Autodesk Inventor part; units mm, degrees
ref_plane "YZ Plane" through (0, 0, 0) normal (1, 0, 0) x (0, 1, 0)
ref_plane "XZ Plane" through (0, 0, 0) normal (0, 1, 0) x (-1, 0, 0)
ref_plane "XY Plane" through (0, 0, 0) normal (0, 0, 1) x (1, 0, 0)
sketch "Sketch1" plane through (0, 0, 0) normal (0, 0, 1) x (1, 0, 0)
  circle A0 centre (0, 0) radius 45
  circle A1 centre (0, 0) radius 10
  dimension "d0" = 90
  dimension "d1" = 20
extrude "Extrusion1" add sketch "Sketch1" along normal blind 10
hole "Hole1" at (0, 0, 0) direction (0, 0, 1) diameter 30 depth 4
sketch "Sketch2" plane through (0, 0, 0) normal (0, 0, -1) x (-1, 0, 0)
  circle A0 centre (0, 35) radius 3.6674
  point P0 (0, 0)
  dimension "d15" = 35
hole "Hole2" at (0, 35, 0) direction (0, 0, 1) diameter 6.6 end through all counterbore diameter 12 counterbore depth 2
chamfer "Chamfer1" distance 4 angle 45 1 edges at (0, 31.7, 10)
pattern_circular "Circular Pattern1" count 5 over 360 about axis through (0, 0, 0) along (0, 0, 1) of "Hole2", "Chamfer1"
properties part number "342-08" material "Titanium"
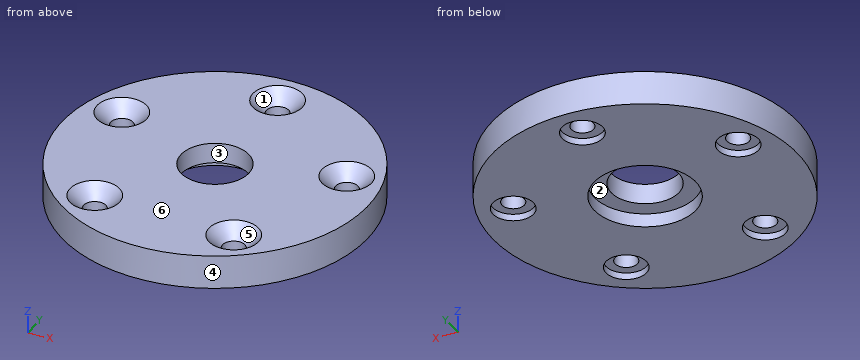
Verification items for the finished model (mm, model axes). Face numbers are marked on the shaded views. A direction names the side the tool comes from. Coordinates: 2 decimals unless noted, no trailing zeros. Order: outer loops, then holes, each group sorted by start corner. A loop starts at its lowest first (then second) coordinate and runs counter-clockwise, first axis right, second up. Notation, with made-up numbers: M 83,60 L 100,60 A36 ccw 100,99 Z; hole C 5,38.5 d1. An arc over 180 degrees is marked long. One line per item, written item: value. Start each with the question number.
Item 1: Sectioned sample at B-B (y = 0). Enter the section's corners in (x, z).
Item 2: Access from +Z, -Z, +X, -X, +Y, -Y to the whole of each face (thin tool, end or side, straight path). Record for the marked faces 1 and 2.
Item 3: Gauge pin test, flat ends, axial feed: pin 1 (6 mm diameter, centred on x = 35.5, y = 9.5, fed in from -Z); pin 2 (7 mm diameter, centred on x = -20.57, y = -28.32, fed in from +Z); pin 3 (5 mm diameter, centred on y = -30.5, z = 2, fed in from -X). Record the tip position at first contact, or that the pin passes through.
Item 4: Sectioned sample at D-D (y = -17). Enter the section's corners in (x, z).
Item 5: Mould release check, pull along X, two halves, no side actions. Record for the marked faces 3, 4, 5 and 6: released by +X, released by -X, zero draft, split by the parting line, or undercut.
Item 6: Sectioned sample at A-A (x = 0). Enter the section's corners in (y, z).
Item 7: Sectioned sample at C-C (y = 35). Enter the section's corners in (x, z), then the cut area to 3 significant figures.
Item 8: Scan lines: probe 1 along Y at (x, z) = (0, 5.75); probe 2 along X at (y, z) = (-32, 8.5); probe 3 along X at (y, z) = (9.5, 2.25). Record each from-to range of solid material in increasing order.
Conclusion:
1. outline: M -45,0 L -15,0 L -15,4 L -10,4 L -10,10 L -45,10 Z; M 10,4 L 15,4 L 15,0 L 45,0 L 45,10 L 10,10 Z
2. face 1: +Z
2. face 2: -Z
3. pin 1: stops at z = 2
3. pin 2: stops at z = 6.21
3. pin 3: stops at x = -35.23
4. outline: M -41.67,0 L 41.67,0 L 41.67,10 L -41.67,10 Z
5. face 3: undercut
5. face 4: split by the parting line
5. face 5: undercut
5. face 6: zero draft
6. outline: M -45,0 L -15,0 L -15,4 L -10,4 L -10,10 L -45,10 Z; M 10,4 L 15,4 L 15,0 L 29,0 L 29,2 L 31.7,2 L 31.7,6 L 27.7,10 L 10,10 Z; M 38.3,2 L 41,2 L 41,0 L 45,0 L 45,10 L 42.3,10 L 38.3,6 Z
7. outline: M -28.28,0 L -6,0 L -6,2 L -3.3,2 L -3.3,6 L -7.3,10 L -28.28,10 Z; M 3.3,2 L 6,2 L 6,0 L 28.28,0 L 28.28,10 L 7.3,10 L 3.3,6 Z
7. area: 473 mm^2
8. probe 1: y = -45 to -10, 10 to 31.7, 38.3 to 45
8. probe 2: x = -31.64 to -25.05, -16.09 to 16.09, 25.05 to 31.64
8. probe 3: x = -43.99 to -36.31, -30.26 to -11.61, 11.61 to 30.26, 36.31 to 43.99
